Work out the finished part from the listing and answer in its coordinate system (mm). A direction names the side the tool comes from. Round coordinates to 2 decimals unless told otherwise and drop trailing zeros. Write each loop counter-clockwise with the first axis right and the second up, starting at its lowest first coordinate (ties: lowest second). Pieces come first, ordered by that corner, then holes.
1. Find section C-C (y = 14.5). Write down the section's boundary in (x, z), and give its area (3 significant figures).
2. Find section B-B (z = 2.4). Write down the section's boundary in (x, y).
3. Find section A-A (x = 0). Write down the section's boundary in (y, z).
4. A tool of negligible diameter and unlimited length cuts with its end or side. For faces 1 (the face through (12, 1, 5)), 2 (the face through (14, 1, 3)), 3 (the face through (0.325, -15.464, 1.146)), 4 (the face through (-10, -15, 3)), 5 (the face through (15, 10, 3)), from which of +Z, -Z, +X, -X, +Y, -Y can it reach the whole face along a straight path? Write none if from no direction.
5. Find section D-D (y = -1). Write down the section's boundary in (x, z).
6. Flat-ended cylindrical pins translate along their axes: pin 1 Ø5 at (x, y) = (9.55, 9.55) entering from +Z; pin 2 Ø1.2 at (y, z) = (-3, 5) entering from -X; pin 3 Ø2 at (x, z) = (-1.5, 2) entering from -Y; pin 4 Ø1.1 at (x, y) = (1, 15.5) entering from +Z. Find the tip coordinate at first contact, or state that the pin passes through.
7. Determine the mould class of faces 6 (the face through (-11, 15, 1)), 7 (the face through (15, -10, 3)), 8 (the face through (0, -12, 5)) for opening direction X: pulls with the +X half, pulls with the -X half, needs draft (parallel to the pull), parting line crosses it, or undercut.
8. Straight lines are drawn through the part: probe 1 along Y at (x, z) = (0, 1.2); probe 2 along X at (y, z) = (-10.5, 4.4); probe 3 along Z at (x, y) = (-13, 3). For each, find the intervals that lie inside material, in ascending order.
```python
from build123d import *

# Parameters (mm, degrees)
SKETCH1_R           = 16
SKETCH1_W           = 30
SKETCH1_H           = 30
BOSS_EXTRUDE1_DEPTH = 6
SKETCH2_R           = 11
CUT_EXTRUDE1_DEPTH  = 10
SKETCH3_R           = 11
CUT_EXTRUDE2_DEPTH  = 4
CUT_EXTRUDE3_DEPTH  = 29
SKETCH5_W           = 8.432235637
SKETCH5_H           = 0.5
SKETCH5_W_2         = 2
CUT_EXTRUDE4_DEPTH  = 29
SKETCH6_R           = 1.5
CUT_EXTRUDE5_DEPTH  = 3


with BuildPart() as part:
    # Sketch1 → Boss-Extrude1 (new body)
    with BuildSketch(Plane.XY):
        Circle(SKETCH1_R)
        Rectangle(SKETCH1_W, SKETCH1_H)
    extrude(amount=BOSS_EXTRUDE1_DEPTH)

    # Sketch2 → Cut-Extrude1 (cut)
    with BuildSketch(Plane.XY.offset(6)):
        Circle(SKETCH2_R)
    extrude(amount=-CUT_EXTRUDE1_DEPTH, mode=Mode.SUBTRACT)

    # Sketch3 → Cut-Extrude2 (cut)
    with BuildSketch(Plane.XY.offset(6)):
        with BuildLine():
            Line((5.567764363, 15), (-5.567764363, 15))
            ThreePointArc((-5.567764363, 15), (-9.057264866, 13.189615353), (-12, 10.583005244))
            Line((-12, 10.583005244), (-12, -10.583005244))
            ThreePointArc((-12, -10.583005244), (-11.313708499, -11.313708499), (-10.583005244, -12))
            Line((-10.583005244, -12), (10.583005244, -12))
            ThreePointArc((10.583005244, -12), (11.313708499, -11.313708499), (12, -10.583005244))
            Line((12, -10.583005244), (12, 10.583005244))
            ThreePointArc((12, 10.583005244), (9.057264866, 13.189615353), (5.567764363, 15))
        make_face()
        Circle(SKETCH3_R, mode=Mode.SUBTRACT)
        with BuildLine():
            ThreePointArc((5.567764363, 15), (0, 16), (-5.567764363, 15))
            Line((-5.567764363, 15), (5.567764363, 15))
        make_face()
        with BuildLine():
            Line((-5.567764363, 15), (-12, 15))
            Line((-12, 15), (-12, 10.583005244))
            ThreePointArc((-12, 10.583005244), (-9.057264866, 13.189615353), (-5.567764363, 15))
        make_face()
        with BuildLine():
            Line((12, 15), (5.567764363, 15))
            ThreePointArc((5.567764363, 15), (9.057264866, 13.189615353), (12, 10.583005244))
            Line((12, 10.583005244), (12, 15))
        make_face()
        with BuildLine():
            Line((12, -12), (12, -10.583005244))
            ThreePointArc((12, -10.583005244), (11.313708499, -11.313708499), (10.583005244, -12))
            Line((10.583005244, -12), (12, -12))
        make_face()
        with BuildLine():
            ThreePointArc((-10.583005244, -12), (-11.313708499, -11.313708499), (-12, -10.583005244))
            Line((-12, -10.583005244), (-12, -12))
            Line((-12, -12), (-10.583005244, -12))
        make_face()
    extrude(amount=-CUT_EXTRUDE2_DEPTH, mode=Mode.SUBTRACT)

    # Sketch4 → Cut-Extrude3 (cut)
    with BuildSketch(Plane(origin=(0, 15, 0), x_dir=(1, 0, 0), z_dir=(0, 1, 0))):
        Polygon((-12, -2), (-14, -2), (-14, -4), (14, -4), (14, -2), (12, -2), align=None)
    extrude(amount=-CUT_EXTRUDE3_DEPTH, mode=Mode.SUBTRACT)

    # Sketch5 → Cut-Extrude4 (cut)
    with BuildSketch(Plane(origin=(0, 15, 0), x_dir=(1, 0, 0), z_dir=(0, 1, 0))):
        Polygon((-14, -2), (-14, -4), (14, -2), (14, -1.5), (-5.567764363, -1.5), (-5.567764363, -2), align=None)
        Polygon((14, -2), (-14, -4), (-12, -4), (-12, -4.5), (14, -4.5), align=None)
        with Locations((-9.783882182, -1.75)):
            Rectangle(SKETCH5_W, SKETCH5_H)
        with Locations((-13, -4.25)):
            Rectangle(SKETCH5_W_2, SKETCH5_H)
    extrude(amount=-CUT_EXTRUDE4_DEPTH, mode=Mode.SUBTRACT)

    # Sketch6 → Cut-Extrude5 (cut)
    with BuildSketch(Plane(origin=(0, 0, 0), x_dir=(-1, 0, 0), z_dir=(0, 0, -1))):
        with Locations((-9.545941546, 9.545941546)):
            Circle(SKETCH6_R)
        with Locations((9.545941546, 9.545941546)):
            Circle(SKETCH6_R)
        with Locations((0, -14)):
            Circle(SKETCH6_R)
    extrude(amount=-CUT_EXTRUDE5_DEPTH, mode=Mode.SUBTRACT)


solid = part.part
```
Worked answers:
1. outline: (-15, 0) - (15, 0) - (15, 6) - (12, 6) - (12, 4.5) - (14, 4.5) - (14, 1.5) - (-14, 1.5) - (-14, 4.5) - (-12, 4.5) - (-12, 6) - (-15, 6) - close
1. area: 60.0 mm2
2. outline: (-15, -15) - (-5.57, -15) arc R16 ccw to (5.57, -15) - (15, -15) - (15, -5.57) arc R16 ccw to (15, 5.57) - (15, 15) - (14, 15) - (14, -14) - (1.5, -14) arc R1.5 cw to (-1.5, -14) - (-14, -14) - (-14, 15) - (-15, 15) - (-15, 5.57) arc R16 ccw to (-15, -5.57) - close
3. outline: (-16, 0) - (-15.5, 0) - (-15.5, 3) - (-14, 3) - (-14, 4.5) - (-12, 4.5) - (-12, 6) - (-16, 6) - close; (-12.5, 0) - (-11, 0) - (-11, 1.5) - (-12.5, 1.5) - close; (11, 0) - (16, 0) - (16, 2) - (15, 2) - (15, 1.5) - (11, 1.5) - close
4. face 1: +Z, +Y
4. face 2: +Y
4. face 3: -Z
4. face 4: +Z, -Z, -X, -Y
4. face 5: +Z, -Z, +X, +Y
5. outline: (-15.97, 0) - (-10.95, 0) - (-10.95, 1.5) - (-14, 1.5) - (-14, 4.5) - (-12, 4.5) - (-12, 6) - (-15.97, 6) - close; (10.95, 0) - (15.97, 0) - (15.97, 6) - (12, 6) - (12, 4.5) - (14, 4.5) - (14, 1.5) - (10.95, 1.5) - close
6. pin 1: stops at z = 6
6. pin 2: stops at x = -15.82
6. pin 3: stops at y = -15.99
6. pin 4: stops at z = 2
7. face 6: needs draft
7. face 7: pulls with the +X half
7. face 8: undercut
8. probe 1: y = -16 to -15.5, -12.5 to -11, 11 to 16
8. probe 2: x = -15 to -14, 14 to 15
8. probe 3: z = 0 to 1.5, 4.5 to 6
